Geometry: final body of the model. Coordinates: model frame, mm. Give positions to 0.01 mm unless a question says otherwise; leave off trailing zeros. Order: outer loops, then holes, each group sorted by start corner. A loop starts at its lowest first (then second) coordinate and runs counter-clockwise, first axis right, second up. Notation, with made-up numbers: M 52.5,48.25 L 88.5,48.25 A31 ccw 88.5,73.25 Z; hole C 78.25,32.25 d5. An arc over 180 degrees is marked long. Use CSV: the item, a comma, the result in double quotes.
```python
from build123d import *

# Parameters (mm, degrees)
SKETCH1_R           = 1.5
SKETCH1_R_2         = 1.499997
SKETCH1_R_3         = 2.54
BOSS_EXTRUDE1_DEPTH = 2.54


with BuildPart() as part:
    # Sketch1 → Boss-Extrude1 (new body)
    with BuildSketch(Plane.XY):
        Polygon((10.998084257, 19.050253087), (-10.998960994, 19.049746903), (-21.99704525, -0.000506184), (-10.998084257, -19.050253087), (10.998960994, -19.049746903), (21.99704525, 0.000506184), align=None)
        with Locations((-12.445999997, -0.000286401)):
            Circle(SKETCH1_R, mode=Mode.SUBTRACT)
        with Locations((12.445999997, 0.000286401)):
            Circle(SKETCH1_R_2, mode=Mode.SUBTRACT)
        Circle(SKETCH1_R_3, mode=Mode.SUBTRACT)
    extrude(amount=BOSS_EXTRUDE1_DEPTH)


solid = part.part
```
1. Pin query (flat end, axial travel): pin 1 Ø3 at (x, y) = (8, -3.5) entering from -Z; pin 2 Ø1 at (y, z) = (-14, 1.5) entering from +X. Return the tip coordinate at first contact, or that it passes through.
Answer:
pin 1,"z = 0"
pin 2,"x = 14.2"
2. Section D-D, the plane x = -17. Return the cut outline in (y, z).
Answer:
outline,"M -8.66,0 L 8.66,0 L 8.66,2.54 L -8.66,2.54 Z"
3. Pull-direction query (X, two-part tool) for faces 1 (the face through (-0.33, 2.52, 1.25)), 2 (the face through (-16.42, 9.66, 1.25)), 3 (the face through (13.832, -0.574, 1.252)), 4 (the face through (5, 0, 2.54)); classes: +X half, -X half, draft (parallel to the pull), parting line (faces both ways), or undercut.
Answer:
face 1,"undercut"
face 2,"-X half"
face 3,"undercut"
face 4,"draft"
4. Line query: line 1 (X direction, y = -1, z = 1.65); line 2 (Y direction, x = 2, z = 1.45). Output: solid intervals per line, ascending.
Answer:
line 1,"-21.42 to -13.56, -11.33 to -2.33, 2.33 to 11.33, 13.56 to 21.42"
line 2,"-19.05 to -1.57, 1.57 to 19.05"
5. Section B-B, the plane z = 1.8. Return the cut outline in (x, y).
Answer:
outline,"M -22,0 L -11,-19.05 L 11,-19.05 L 22,0 L 11,19.05 L -11,19.05 Z; hole C -12.45,0 d3; hole C 0,0 d5.08; hole C 12.45,0 d3"
6. Section A-A, the plane x = 0. Return the cut outline in (y, z), plus the area to 3 significant figures.
Answer:
outline,"M -19.05,0 L -2.54,0 L -2.54,2.54 L -19.05,2.54 Z; M 2.54,0 L 19.05,0 L 19.05,2.54 L 2.54,2.54 Z"
area,"83.9 mm2"
7. Section C-C, the plane y = 16.5. Return the cut outline in (x, z), plus the area to 3 significant figures.
Answer:
outline,"M -12.47,0 L 12.47,0 L 12.47,2.54 L -12.47,2.54 Z"
area,"63.4 mm2"
